```python
from build123d import *

# Parameters (mm, degrees)
CHAMFER1_SIZE      = 1
SKETCH2_R          = 2.5
CUT_EXTRUDE1_DEPTH = 97.115975922
CUT_EXTRUDE2_DEPTH = 4


with BuildPart() as part:
    # Sketch1 → Revolve1 (revolve)
    with BuildSketch(Plane.XY, mode=Mode.PRIVATE) as revolve1_sk:
        Polygon((-92.26744186, 0), (-92.26744186, 10), (-77.26744186, 10), (-77.26744186, 14), (-69.26744186, 14), (-69.26744186, 12), (-31.26744186, 12), (-31.26744186, 10), (18.73255814, 10), (18.73255814, 9), (53.73255814, 9), (53.73255814, 0), align=None)
    revolve(revolve1_sk.sketch.rotate(Axis((-99.418604651, 0, 0), (1, 0, 0)), 90), axis=Axis((-99.418604651, 0, 0), (1, 0, 0)))

    # Chamfer1
    chamfer1_edges = [part.edges().sort_by_distance(p)[0] for p in [
        (-92.26744186, 0, -10),
        (53.73255814, 0, -9),
    ]]
    chamfer(chamfer1_edges, length=CHAMFER1_SIZE)

    # Sketch2 → Cut-Extrude1 (cut, through all)
    with BuildSketch(Plane(origin=(0, 9, 0), x_dir=(1, 0, 0), z_dir=(0, 1, 0))):
        with Locations(Location((43.73255814, 0, 0), (0, 0, 270))):
            Circle(SKETCH2_R)
    extrude(amount=-CUT_EXTRUDE1_DEPTH, mode=Mode.SUBTRACT)

    # Sketch3 → Cut-Extrude2 (cut)
    with BuildSketch(Plane(origin=(0, 12, 0), x_dir=(1, 0, 0), z_dir=(0, 1, 0))):
        with BuildLine():
            Line((-59.26744186, 4), (-39.26744186, 4))
            ThreePointArc((-39.26744186, 4), (-35.26744186, 0), (-39.26744186, -4))
            Line((-39.26744186, -4), (-59.26744186, -4))
            ThreePointArc((-59.26744186, -4), (-63.26744186, 0), (-59.26744186, 4))
        make_face()
    extrude(amount=-CUT_EXTRUDE2_DEPTH, mode=Mode.SUBTRACT)


solid = part.part
```
Source: CAD feature listing. Evaluate the final solid. Frame: model axes, mm. A direction names the side the tool comes from. Coordinates: 2 decimals unless noted, no trailing zeros. Order: outer loops, then holes, each group sorted by start corner. A loop starts at its lowest first (then second) coordinate and runs counter-clockwise, first axis right, second up. Notation, with made-up numbers: M 72.5,-7 L 104.5,-7 A34 ccw 104.5,28 Z; hole C 65.25,69 d4. An arc over 180 degrees is marked long. Write each question's results on one line, items separated by ' | '. Start each with the question number.
1) Line query: line 1 (X direction, y = -3.25, z = 0); line 2 (Z direction, x = -55, y = 0.25); line 3 (X direction, y = 10.25, z = 2.5). Output: solid intervals per line, ascending. Write a range as from..to.
2) Draft query along X for faces 1 (the face through (-35.27, 10.03, -0.09)), 2 (the face through (-84, 0, -10)), 3 (the face through (-49, 10, 4)), 4 (the face through (-31.267, -9, -5)). Return one class per face: released by +X, released by -X, zero draft, split by the parting line, or undercut.
3) Access query for faces 5 (the face through (-63.266, 10.028, 0.088)), 6 (the face through (35.971, -2.703, 8.584)), 7 (the face through (-77.267, -10, 3)). Directions: +Z, -Z, +X, -X, +Y, -Y. A direction counts if a zero-diameter tool reaches every point of the face in a straight line with its end or side. Return the directions, or none.
4) Section query D-D (x = -82.5). Return the cut outline in (y, z).
5) Section query B-B (y = 0). Return the cut outline in (x, z).
6) Contact query for flat-ended pins moving along their axis: pin 1 Ø8 at (x, z) = (-70.5, -9) entering from +Y; pin 2 Ø8 at (x, z) = (-2, 8.5) entering from +Y; pin 3 Ø2 at (x, z) = (-23, 0.5) entering from +Y; pin 4 Ø10 at (x, z) = (-67.5, 0) entering from -Y. Output: stop coordinate, or through.
7) Section query C-C (x = -52.5). Return the cut outline in (y, z).
Answers:
1) line 1: x = -92.27..41.23, 46.23..53.73 | line 2: z = -12..12 | line 3: x = -77.27..-62.39, -36.14..-31.27
2) face 1: undercut | face 2: zero draft | face 3: undercut | face 4: released by +X
3) face 5: +Y | face 6: +X | face 7: -X
4) outline: C 0,0 d20
5) outline: M -92.27,-9 L -91.27,-10 L -77.27,-10 L -77.27,-14 L -69.27,-14 L -69.27,-12 L -31.27,-12 L -31.27,-10 L 18.73,-10 L 18.73,-9 L 52.73,-9 L 53.73,-8 L 53.73,8 L 52.73,9 L 18.73,9 L 18.73,10 L -31.27,10 L -31.27,12 L -69.27,12 L -69.27,14 L -77.27,14 L -77.27,10 L -91.27,10 L -92.27,9 Z; hole C 43.73,0 d5
6) pin 1: stops at y = 13.08 | pin 2: stops at y = 8.93 | pin 3: stops at y = 10 | pin 4: stops at y = -14
7) outline: M 8,-4 L 8,4 L 11.31,4 A12 ccw long 11.31,-4 Z
